Geometry: final body of the model. Coordinates: model frame, mm. Face numbers are marked on the shaded views. A direction names the side the tool comes from. Coordinates: 2 decimals unless noted, no trailing zeros. Loops run counter-clockwise (first coordinate to the right, second up) from the corner with the lowest first, then second, coordinate; pieces in that order, holes last. Notation, with made-up numbers: (20.25, 7) - (38.25, 7) arc R20 cw to (38.25, 40) - close; hole circle Ø7 at (31, 6.5). An arc over 180 degrees is marked (long way). Put each result on its own line as item: value. Start each with the question number.
1) Section B-B on z = 0.75. Output: boundary loops of the cut face in (x, y).
2) Section D-D on x = 6.5. Output: boundary loops of the cut face in (y, z).
3) Material intervals for line 1 along Y through (x, z) = (3.5, 0.05); line 2 along Z through (x, y) = (3.8, -41.5); line 3 along Z through (x, y) = (2.5, -24), sorted ascending. Write a range as from..to.
4) Reachability of the marked faces 1, 2, 3, 4 and 5 from +Z, -Z, +X, -X, +Y, -Y: full face, straight path, thin tool, end or side. Return the list, or none.
5) Contact query for flat-ended pins moving along their axis: pin 1 Ø4 at (x, z) = (1.5, -3) entering from -Y; pin 2 Ø2 at (y, z) = (-39.5, 1) entering from +X; pin 3 Ø2.5 at (x, y) = (3.5, -3) entering from -Z. Output: stop coordinate, or through.
6) Section A-A on x = 3.5. Count the separate pieces of the cut face and the enclosed holes in it, and give its area (3 significant figures).
7) Section C-C on y = -9.5. Output: boundary loops of the cut face in (x, z), and give its area (3 significant figures).
8) Draft query along Y for the marked faces 6, 7, 8 and 9. Return one class per face: +Y half, -Y half, draft (parallel to the pull), parting line (faces both ways), or undercut.
```python
from build123d import *

# Parameters (mm, degrees)
SKETCH1_R           = 1
BOSS_EXTRUDE1_DEPTH = 1.5
BOSS_EXTRUDE2_DEPTH = 3.5
FILLET1_R           = 2
FILLET2_R           = 2
FILLET4_R           = 3.5
SKETCH2_R           = 1.5
CUT_EXTRUDE1_DEPTH  = 7


with BuildPart() as part:
    # Sketch1 → Boss-Extrude1 (new, symmetric)
    with BuildSketch(Plane.XY):
        with BuildLine():
            Line((3, 0), (4, 0))
            ThreePointArc((4, 0), (6.121320344, -0.878679656), (7, -3))
            Line((7, -3), (7, -27))
            ThreePointArc((7, -27), (6.121320344, -29.121320344), (4, -30))
            Line((4, -30), (3, -30))
            ThreePointArc((3, -30), (0.878679656, -29.121320344), (0, -27))
            Line((0, -27), (0, -3))
            ThreePointArc((0, -3), (0.878679656, -0.878679656), (3, 0))
        make_face()
        with Locations((3.5, -3)):
            Circle(SKETCH1_R, mode=Mode.SUBTRACT)
    extrude(amount=BOSS_EXTRUDE1_DEPTH, both=True)

    # Sketch1<3> → Boss-Extrude2 (add, symmetric)
    with BuildSketch(Plane.XY):
        Polygon((4, -30), (3, -30), (2, -30), (2, -45), (5, -45), (5, -30), align=None)
    extrude(amount=BOSS_EXTRUDE2_DEPTH, both=True)

    # Fillet1
    fillet1_edges = [part.edges().sort_by_distance(p)[0] for p in [
        (3.5, -30, 3.5),
    ]]
    fillet(fillet1_edges, radius=FILLET1_R - 0.0001)  # a hair under: the kernel refuses the full size

    # Fillet2
    fillet2_edges = [part.edges().sort_by_distance(p)[0] for p in [
        (3.5, -30, -3.5),
    ]]
    fillet(fillet2_edges, radius=FILLET2_R - 0.0001)  # a hair under: the kernel refuses the full size

    # Fillet4
    fillet4_edges = [part.edges().sort_by_distance(p)[0] for p in [
        (3.5, -45, 3.5),
        (3.5, -45, -3.5),
    ]]
    fillet(fillet4_edges, radius=FILLET4_R - 0.0001)  # a hair under: the kernel refuses the full size

    # Sketch2 → Cut-Extrude1 (cut)
    with BuildSketch(Plane(origin=(5, 0, 0), x_dir=(0, 0, -1), z_dir=(1, 0, 0))):
        with Locations(Location((0, -41.5, 0), (0, 0, 90))):
            Circle(SKETCH2_R)
    extrude(amount=-CUT_EXTRUDE1_DEPTH, mode=Mode.SUBTRACT)


solid = part.part
```
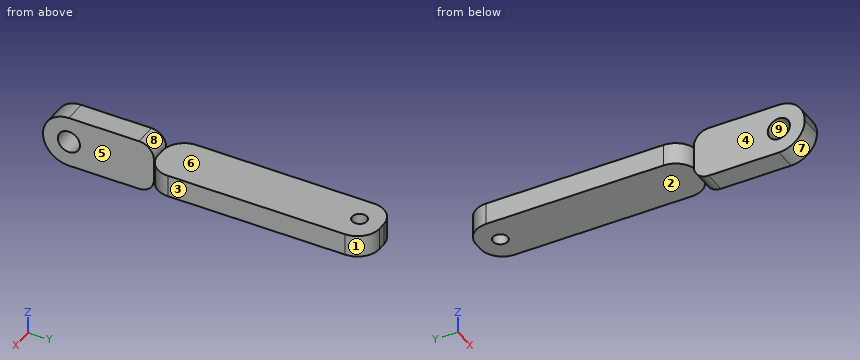
Answer block:
1. outline: (0, -27) arc R3 ccw to (3, -30) - (2, -30) - (2, -40.2) - (5, -40.2) - (5, -30) - (4, -30) arc R3 ccw to (7, -27) - (7, -3) arc R3 ccw to (4, 0) - (3, 0) arc R3 ccw to (0, -3) - close; (2, -44.92) - (5, -44.92) - (5, -42.8) - (2, -42.8) - close; hole circle Ø2 at (3.5, -3)
2. outline: (-28.66, -1.5) - (-1.34, -1.5) - (-1.34, 1.5) - (-28.66, 1.5) - close
3. line 1: y = -45..-43, -40..-4, -2..0
3. line 2: z = -3.5..-1.5, 1.5..3.5
3. line 3: z = -1.5..1.5
4. face 1: +Z, -Z, +X, +Y
4. face 2: -Z, +X, -X, +Y
4. face 3: +Z, -Z, +X, +Y, -Y
4. face 4: +Z, -Z, -X, -Y
4. face 5: +Z, -Z, +X, -Y
5. pin 1: stops at y = -44.83
5. pin 2: stops at x = 5
5. pin 3: stops at z = -1.5
6. separate pieces: 2
6. enclosed holes: 1
6. area: 175 mm²
7. outline: (0, -1.5) - (7, -1.5) - (7, 1.5) - (0, 1.5) - close
7. area: 21.0 mm²
8. face 6: draft
8. face 7: -Y half
8. face 8: +Y half
8. face 9: undercut
